Work out the finished part from the listing and answer in its coordinate system (mm). Round coordinates to 2 decimals unless told otherwise and drop trailing zeros. Order: outer loops, then holes, each group sorted by start corner. A loop starts at its lowest first (then second) coordinate and runs counter-clockwise, first axis right, second up. Notation, with made-up numbers: (-0.75, 9) - (11.25, 9) arc R22 ccw to (11.25, 39) - close; hole circle Ø10 at (65, 51.5). An arc over 180 degrees is marked (long way). Use CSV: the item, a comma, the result in double quotes.
from build123d import *

# Parameters (mm, degrees)
TOP_AND_BOTTOM_R              = 1.5
TOP_AND_BOTTOM_R_2            = 2.5
TOP_AND_BOTTOM_W              = 12
TOP_AND_BOTTOM_H              = 12
TOP_AND_BOTTOM_W_2            = 7.5
TOP_AND_BOTTOM_H_2            = 14
TOP_AND_BOTTOM_EXTRUDED_DEPTH = 3


with BuildPart() as part:
    # Top and Bottom → Top and Bottom Extruded (new body)
    with BuildSketch(Plane(origin=(0, 0, 0), x_dir=(1, 0, 0), z_dir=(0, 1, 0))):
        Polygon((32, 60), (48, 60), (48, 57), (64, 57), (64, 60), (80, 60), (80, 40), (77, 40), (77, 20), (80, 20), (80, 0), (64, 0), (64, 3), (48, 3), (48, 0), (32, 0), (32, 3), (16, 3), (16, 0), (0, 0), (0, 20), (3, 20), (3, 40), (0, 40), (0, 60), (16, 60), (16, 57), (32, 57), align=None)
        with Locations(Location((28.75, 37.75, 0), (0, 0, 270))):
            Circle(TOP_AND_BOTTOM_R, mode=Mode.SUBTRACT)
        with Locations(Location((46.75, 37.75, 0), (0, 0, 270))):
            Circle(TOP_AND_BOTTOM_R, mode=Mode.SUBTRACT)
        with Locations(Location((64.75, 37.75, 0), (0, 0, 270))):
            Circle(TOP_AND_BOTTOM_R, mode=Mode.SUBTRACT)
        with Locations(Location((13, 37.75, 0), (0, 0, 270))):
            Circle(TOP_AND_BOTTOM_R_2, mode=Mode.SUBTRACT)
        with Locations((46.75, 25.75)):
            Rectangle(TOP_AND_BOTTOM_W, TOP_AND_BOTTOM_H, mode=Mode.SUBTRACT)
        with Locations((28.75, 25.75)):
            Rectangle(TOP_AND_BOTTOM_W, TOP_AND_BOTTOM_H, mode=Mode.SUBTRACT)
        with Locations((64.75, 25.75)):
            Rectangle(TOP_AND_BOTTOM_W, TOP_AND_BOTTOM_H, mode=Mode.SUBTRACT)
        with Locations((13, 26.75)):
            Rectangle(TOP_AND_BOTTOM_W_2, TOP_AND_BOTTOM_H_2, mode=Mode.SUBTRACT)
    extrude(amount=TOP_AND_BOTTOM_EXTRUDED_DEPTH)


solid = part.part
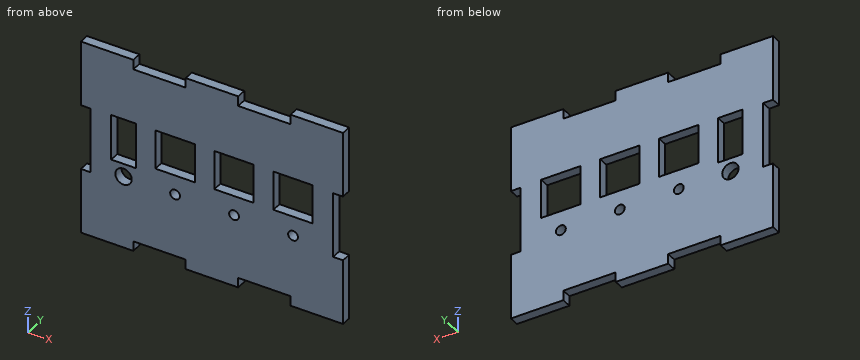
(1) Each of these flat-tipped pins is pushed along its axis until it touches: pin 1 (1.5 mm diameter, centred on y = 2, z = -27, fed in from -X); pin 2 (1 mm diameter, centred on x = 20, y = 0.5, fed in from -Z); pin 3 (1.5 mm diameter, centred on y = 1.5, z = -24, fed in from +X). Where does it stop, or does it pass through?
Findings below:
pin 1,"stops at x = 3"
pin 2,"stops at z = -57"
pin 3,"stops at x = 77"
(2) Find section A-A (x = 28.75). Determine the outline of the cut face in (y, z).
Findings below:
outline,"(0, -57) - (3, -57) - (3, -39.25) - (0, -39.25) - close; (0, -36.25) - (3, -36.25) - (3, -31.75) - (0, -31.75) - close; (0, -19.75) - (3, -19.75) - (3, -3) - (0, -3) - close"
(3) Find section B-B (z = -23). Determine the outline of the cut face in (x, y), and give its area (3 significant figures).
Findings below:
outline,"(3, 0) - (9.25, 0) - (9.25, 3) - (3, 3) - close; (16.75, 0) - (22.75, 0) - (22.75, 3) - (16.75, 3) - close; (34.75, 0) - (40.75, 0) - (40.75, 3) - (34.75, 3) - close; (52.75, 0) - (58.75, 0) - (58.75, 3) - (52.75, 3) - close; (70.75, 0) - (77, 0) - (77, 3) - (70.75, 3) - close"
area,"91.5 mm²"
(4) Find section D-D (x = 13). Determine the outline of the cut face in (y, z).
Findings below:
outline,"(0, -60) - (3, -60) - (3, -40.25) - (0, -40.25) - close; (0, -35.25) - (3, -35.25) - (3, -33.75) - (0, -33.75) - close; (0, -19.75) - (3, -19.75) - (3, 0) - (0, 0) - close"
(5) Find the intervals of material crossed by L1, parallel to X at y = 2.1, z = -37.75; L2, parallel to X at y = 0.9, z = -30.5; L3, parallel to Z at x = 63.5, y = 0.9, in increasing order. Write a range as from..to.
Findings below:
L1,"x = 3..10.5, 15.5..27.25, 30.25..45.25, 48.25..63.25, 66.25..77"
L2,"x = 3..9.25, 16.75..22.75, 34.75..40.75, 52.75..58.75, 70.75..77"
L3,"z = -57..-38.58, -36.92..-31.75, -19.75..-3"
(6) Find section C-C (x = 68.5). Determine the outline of the cut face in (y, z).
Findings below:
outline,"(0, -60) - (3, -60) - (3, -31.75) - (0, -31.75) - close; (0, -19.75) - (3, -19.75) - (3, 0) - (0, 0) - close"
